```python
from build123d import *

# Parameters (mm, degrees)
SKETCH1_W                          = 25.4
SKETCH1_H                          = 12.7
STOCK_DEPTH                        = 79.375
SKETCH2_W                          = 12.7
SKETCH2_H                          = 53.975
CUTOUT_DEPTH                       = 85.302079601
FILLET1_R                          = 6.35
F_1_4_0_25_DIAMETER_HOLE1_D        = 6.35
MOUNTING_HOLES_ONE_SIDE_AT_2_COUNT = 2
MOUNTING_HOLES_ONE_SIDE_AT_2_PITCH = 15.24


with BuildPart() as part:
    # Sketch1 → Stock (new body)
    with BuildSketch(Plane(origin=(0, 0, 0), x_dir=(1, 0, 0), z_dir=(0, 1, 0))):
        with Locations((12.7, 6.35)):
            Rectangle(SKETCH1_W, SKETCH1_H)
    extrude(amount=STOCK_DEPTH)

    # Sketch2 → Cutout (cut, through all)
    with BuildSketch(Plane.XY):
        with Locations((6.35, 39.6875)):
            Rectangle(SKETCH2_W, SKETCH2_H)
    extrude(amount=-CUTOUT_DEPTH, mode=Mode.SUBTRACT)

    # Fillet1
    fillet1_edges = [part.edges().sort_by_distance(p)[0] for p in [
        (12.7, 66.675, -6.35),
        (12.7, 12.7, -6.35),
    ]]
    fillet(fillet1_edges, radius=FILLET1_R)

    # 1/4 (0.25) Diameter Hole1 (through all)
    with Locations(Plane.ZY.offset(-12.7)):
        with Locations((-6.35, 39.6875)):
            Hole(F_1_4_0_25_DIAMETER_HOLE1_D / 2)

    # Sketch8 → Mounting Holes One Side (revolve, cut)
    with BuildSketch(Plane(origin=(5.08, 79.375, -6.35), x_dir=(0, 0, 1), z_dir=(1, 0, 0))):
        Polygon((0, 0), (0, 13.840824014), (1.89865, 12.7), (1.89865, 0), align=None)
    mounting_holes_one_side = revolve(axis=Axis((5.08, 85.725, -6.35), (0, -1, 0)), mode=Mode.SUBTRACT)

    # Mounting Holes One Side at 2: Mounting Holes One Side ×2
    with Locations(*[(i * MOUNTING_HOLES_ONE_SIDE_AT_2_PITCH, 0, 0) for i in range(1, MOUNTING_HOLES_ONE_SIDE_AT_2_COUNT)]):
        add(mounting_holes_one_side, mode=Mode.SUBTRACT)

    # Mounting Holes: Mounting Holes One Side across plane
    add(mounting_holes_one_side.mirror(Plane(origin=(0, 39.6875, 0), x_dir=(0, 0, 1), z_dir=(0, -1, 0))), mode=Mode.SUBTRACT)

    # Mounting Holes copy 1 sketch → Mounting Holes copy 1 (revolve, cut)
    with BuildSketch(Plane(origin=(20.32, 0, -6.35), x_dir=(0, 0, 1), z_dir=(1, 0, 0))):
        Polygon((0, 0), (0, -13.840824014), (1.89865, -12.7), (1.89865, 0), align=None)
    revolve(axis=Axis((20.32, -6.35, -6.35), (0, -1, 0)), mode=Mode.SUBTRACT)


solid = part.part
```
CAD build for the part. Positions are in the model's coordinates, mm. A direction names the side the tool comes from. Round coordinates to 2 decimals unless told otherwise and drop trailing zeros. Write each loop counter-clockwise with the first axis right and the second up, starting at its lowest first coordinate (ties: lowest second). Pieces come first, ordered by that corner, then holes.
Item 1: Drop flat-ended pins along their axis: pin 1 Ø6.5 at (y, z) = (33.5, -7.5) entering from -X; pin 2 Ø2.5 at (x, z) = (20.32, -6.35) entering from -Y; pin 3 Ø5 at (y, z) = (39.69, -6.35) entering from -X. Give the stop position or say it passes through.
Filled in:
pin 1: stops at x = 12.7
pin 2: stops at y = 13.09
pin 3: passes through
Item 2: Band-saw the part on D-D on y = 22.5. Write the cut outline in (x, z).
Filled in:
outline: (12.7, -12.7) - (25.4, -12.7) - (25.4, 0) - (12.7, 0) - close
Item 3: Drill centre lines: L1, parallel to X at y = 70.5, z = -6.35; L2, parallel to Z at x = 5.08, y = 6; L3, parallel to Y at x = 4, z = -1 (3 decimals). Where is each one in solid material? Low to high.
Filled in:
L1: x = 0 to 3.18, 6.98 to 18.42, 22.22 to 25.4
L2: z = -12.7 to -8.25, -4.45 to 0
L3: y = 0 to 12.7, 66.675 to 79.375
Item 4: Band-saw the part on B-B on y = 5.5. Write the cut outline in (x, z), then the cut area to 3 significant figures.
Filled in:
outline: (0, -12.7) - (25.4, -12.7) - (25.4, 0) - (0, 0) - close; hole circle Ø3.8 at (5.08, -6.35); hole circle Ø3.8 at (20.32, -6.35)
area: 300 mm2
Item 5: Tool access for faces 4 (the flat face through (3, 12.7, -6)), 5 (the cylindrical face through (22.174, 73.114, -6.762)), 6 (the flat face through (25.4, 39, -10)), 7 (the cylindrical face through (22.174, 6.261, -6.762)): list every direction of +Z, -Z, +X, -X, +Y, -Y with a clear straight run to the whole face (end or side of a thin tool).
Filled in:
face 4: +Z, -Z, -X
face 5: +Y
face 6: +Z, -Z, +X, +Y, -Y
face 7: -Y
Item 6: Mould opens along Z. For faces 1 (the flat face through (13, 0, -6)), 2 (the flat face through (15, 39, -12.7)), 3 (the conical face through (20.221, 13.643, -6.035)) say: released by +Z, released by -Z, zero draft, split by the parting line, or undercut.
Filled in:
face 1: zero draft
face 2: released by -Z
face 3: undercut
Item 7: Band-saw the part on A-A on x = 5.08. Write the cut outline in (y, z) (3 decimals), then the cut area to 3 significant figures.
Filled in:
outline: (0, -12.7) - (12.7, -12.7) - (12.7, -8.249) - (0, -8.249) - close; (0, -4.451) - (12.7, -4.451) - (12.7, 0) - (0, 0) - close; (66.675, -12.7) - (79.375, -12.7) - (79.375, -8.249) - (66.675, -8.249) - close; (66.675, -4.451) - (79.375, -4.451) - (79.375, 0) - (66.675, 0) - close
area: 226 mm2
